Build history of the part. All positions in model axes, mm. Face numbers are marked on the shaded views. A direction names the side the tool comes from. Round coordinates to 2 decimals unless told otherwise and drop trailing zeros. Write each loop counter-clockwise with the first axis right and the second up, starting at its lowest first coordinate (ties: lowest second). Pieces come first, ordered by that corner, then holes. Notation, with made-up numbers: (71, 23.5) -> (125, 23.5) arc R7 ccw to (125, 35.5) -> close; hole circle Ø6 at (-31, -28). An arc over 180 degrees is marked (long way). Answer in a Markdown table with one row per item.
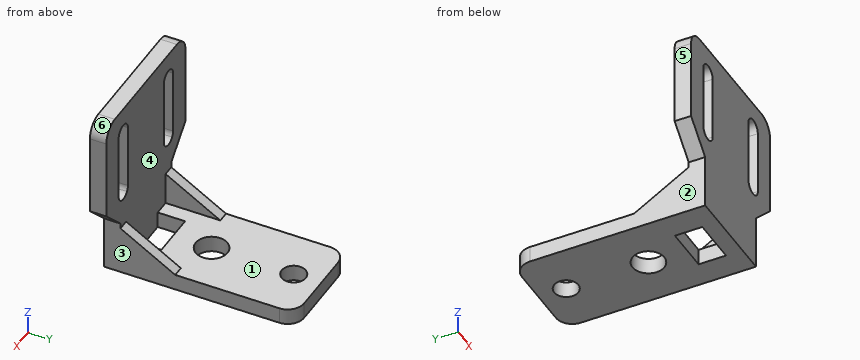
```python
from build123d import *

# Parameters (mm, degrees)
F0_W     = 18
F0_H     = 35
F0_W_2   = 8.4
F0_H_2   = 5
F0_R     = 2.9
F0_R_2   = 2.2
F1_DEPTH = 3
F2_W     = 18
F2_H     = 7
F3_DEPTH = 3
F5_START = 7
F5_DEPTH = 2
F6_START = -7
F6_DEPTH = 2
F7_R     = 3


with BuildPart() as f1:
    # F0 (on Top) → F1 (new body)
    with BuildSketch(Plane.XY):
        Rectangle(F0_W, F0_H)
        with Locations((0, -12)):
            Rectangle(F0_W_2, F0_H_2, mode=Mode.SUBTRACT)
        with Locations((0, -2.5)):
            Circle(F0_R, mode=Mode.SUBTRACT)
        with Locations((0, 12.5)):
            Circle(F0_R_2, mode=Mode.SUBTRACT)
    extrude(amount=F1_DEPTH)

    # F2 (on face) → F3 (join)
    with BuildSketch(Plane.XZ.offset(17.5)):
        with Locations((0, 6.5)):
            Rectangle(F2_W, F2_H)
        with BuildLine():
            Line((-14, 15), (-9, 10))
            Line((-9, 10), (9, 10))
            Line((9, 10), (14, 15))
            Line((14, 15), (9.3124404748, 15))
            ThreePointArc((9.3124404748, 15), (8, 14.35), (6.6875595252, 15))
            Line((6.6875595252, 15), (-6.6875595252, 15))
            ThreePointArc((-6.6875595252, 15), (-8, 14.35), (-9.3124404748, 15))
            Line((-9.3124404748, 15), (-14, 15))
        make_face()
        with BuildLine():
            Line((-14, 33), (-14, 15))
            Line((-14, 15), (-9.3124404748, 15))
            ThreePointArc((-9.3124404748, 15), (-9.5633340627, 15.4722816961), (-9.65, 16))
            Line((-9.65, 16), (-9.65, 28))
            ThreePointArc((-9.65, 28), (-8, 29.65), (-6.35, 28))
            Line((-6.35, 28), (-6.35, 16))
            ThreePointArc((-6.35, 16), (-6.4366659373, 15.4722816961), (-6.6875595252, 15))
            Line((-6.6875595252, 15), (6.6875595252, 15))
            ThreePointArc((6.6875595252, 15), (6.4366659373, 15.4722816961), (6.35, 16))
            Line((6.35, 16), (6.35, 28))
            ThreePointArc((6.35, 28), (8, 29.65), (9.65, 28))
            Line((9.65, 28), (9.65, 16))
            ThreePointArc((9.65, 16), (9.5633340627, 15.4722816961), (9.3124404748, 15))
            Line((9.3124404748, 15), (14, 15))
            Line((14, 15), (14, 33))
            Line((14, 33), (-14, 33))
        make_face()
    extrude(amount=-F3_DEPTH)

    # F4 (on Right) → F5 (join)
    with BuildSketch(Plane.YZ.offset(F5_START)):
        Polygon((-4.5, 3), (-14.5, 9), (-14.5, 3), align=None)
    extrude(amount=F5_DEPTH)

    # F4 (on Right) → F6 (join)
    with BuildSketch(Plane.YZ.offset(F6_START)):
        Polygon((-4.5, 3), (-14.5, 9), (-14.5, 3), align=None)
    extrude(amount=-F6_DEPTH)

    # F7
    f7_edges = [f1.edges().sort_by_distance(p)[0] for p in [
        (-14, -16, 33),
        (14, -16, 33),
        (9, 17.5, 1.5),
        (-9, 17.5, 1.5),
    ]]
    fillet(f7_edges, radius=F7_R)


solid = f1.part
```
Q1. Saw through at A-A on y = 12.5. Write the cut outline in (x, z).
A:
| item | result |
|---|---|
| outline | (-9, 0) -> (-2.2, 0) -> (-2.2, 3) -> (-9, 3) -> close; (2.2, 0) -> (9, 0) -> (9, 3) -> (2.2, 3) -> close |
Q2. Wall check: line 1 (Y direction, x = 0, z = 1.4); line 2 (Y direction, x = 11.25, z = 21); line 3 (Z direction, x = -7.25, y = 12.5). Give the ranges that are in metal, low to high. Write a range as [from, to].
A:
| item | result |
|---|---|
| line 1 | [-17.5, -14.5], [-9.5, -5.4], [0.4, 10.3], [14.7, 17.5] |
| line 2 | [-17.5, -14.5] |
| line 3 | [0, 3] |
Q3. Saw through at B-B on z = 26. Write the cut outline in (x, y), plus the area to 3 significant figures.
A:
| item | result |
|---|---|
| outline | (-14, -17.5) -> (-9.65, -17.5) -> (-9.65, -14.5) -> (-14, -14.5) -> close; (-6.35, -17.5) -> (6.35, -17.5) -> (6.35, -14.5) -> (-6.35, -14.5) -> close; (9.65, -17.5) -> (14, -17.5) -> (14, -14.5) -> (9.65, -14.5) -> close |
| area | 64.2 mm² |
Q4. Saw through at D-D on y = -10.5. Write the cut outline in (x, z), plus the area to 3 significant figures.
A:
| item | result |
|---|---|
| outline | (-9, 0) -> (-4.2, 0) -> (-4.2, 3) -> (-7, 3) -> (-7, 6.6) -> (-9, 6.6) -> close; (4.2, 0) -> (9, 0) -> (9, 6.6) -> (7, 6.6) -> (7, 3) -> (4.2, 3) -> close |
| area | 43.2 mm² |
Q5. Drop flat-ended pins along their axis: P1, Ø8, axis at y = -11, z = 27, coming from the -X side; P2, Ø8, axis at y = 4, z = 5.5, coming from the -X side; P3, Ø5, axis at x = -5, y = -3.5, coming from the +Z side; P4, Ø4, axis at x = 0, y = 12.5, coming from the +Z side. Give the stop position or say it passes through.
A:
| item | result |
|---|---|
| P1 | x = -14 |
| P2 | x = -9 |
| P3 | z = 3.3 |
| P4 | through |
Q6. Saw through at C-C on x = -8. Write the cut outline in (y, z), plus the area to 3 significant figures.
A:
| item | result |
|---|---|
| outline | (-17.5, 0) -> (16.74, 0) -> (16.74, 3) -> (-4.5, 3) -> (-14.5, 9) -> (-14.5, 14.35) -> (-17.5, 14.35) -> close; (-17.5, 29.65) -> (-14.5, 29.65) -> (-14.5, 33) -> (-17.5, 33) -> close |
| area | 177 mm² |
Q7. Which spindle directions (+Z, -Z, +X, -X, +Y, -Y) get a long thin tool onto all of the face, cutting with end or side? Do the marked faces 1, 2 and 3. Say none if no direction does.
A:
| item | result |
|---|---|
| face 1 | +Z, +Y |
| face 2 | -Z, -X, +Y, -Y |
| face 3 | -Z, +X, +Y, -Y |
Q8. Two-plate mould, pull along X, no slides. Class the marked faces 4, 5 and 6: released by +X, released by -X, zero draft, split by the parting line, or undercut.
A:
| item | result |
|---|---|
| face 4 | undercut |
| face 5 | released by -X |
| face 6 | released by +X |
